Design review of the part built by this model. Coordinates are the model's own, in mm. A direction names the side the tool comes from. Coordinates: 2 decimals unless noted, no trailing zeros. Loops run counter-clockwise (first coordinate to the right, second up) from the corner with the lowest first, then second, coordinate; pieces in that order, holes last. Notation, with made-up numbers: (-3.75, -32.5) - (48.25, -32.5) arc R4 ccw to (48.25, -25.5) - close; hole circle Ø6 at (30, -12). An arc over 180 degrees is marked (long way). Use one line per item in the form item = value. Start each with the question number.
(1) Add section B-B (y = 11.75). State the section outline as (x, z) points.
(2) Clearance check with flat-ended pins moving along their axes: pin 1 Ø1.5 at (x, z) = (19.5, 19) entering from +Y; pin 2 Ø1 at (x, z) = (39, 16) entering from +Y. State where each tip first meets the part, or that it passes through.
(3) Add section D-D (z = 18.5). State the section outline as (x, y) points.
(4) The part is to be moulded in two halves that separate along Z. For faces 1 (the face through (-1, 0, -21)), 2 (the face through (-28, 2, 0)), say which applies: pulls with the +Z half, pulls with the -Z half, needs draft (parallel to the pull), parting line crosses it, or undercut.
(5) Add section A-A (z = 0). State the section outline as (x, y) points.
(6) Tool access review of faces 3 (the face through (-22, 2, 0)), 4 (the face through (-56, 14, -44)), 5 (the face through (57, 4, -43)): name each direction out of +Z, -Z, +X, -X, +Y, -Y from which nothing blocks a thin tool from reaching the whole face with its end or side.
(7) Add section C-C (x = 25). State the section outline as (y, z) points.
(8) For L1, parallel to X at y = 5.5, z = 18.5; L2, parallel to X at y = 2.25, z = 0; L3, parallel to Z at x = 56, y = 2.8, list the stretches that pass through material, from the lowest coordinate up.
```python
from build123d import *
from build123d.topology import SkipClean

# Parameters (mm, degrees)
SKETCH1_W               = 31
SKETCH1_H               = 26
SKETCH1_R               = 2.5
SKETCH1_R_2             = 5
BOSS_EXTRUDE1_DEPTH     = 4
FILLET1_R               = 4
BOSS_EXTRUDE2_START     = 10
SKETCH2_R               = 4
BOSS_EXTRUDE2_DEPTH     = 10
MIRROR2_START           = 10
MIRROR2_COPY_1_SKETCH_R = 4
MIRROR2_COPY_1_DEPTH    = 10
SKETCH3_R               = 1.75
CUT_EXTRUDE1_DEPTH      = 4
MIRROR4_COPY_1_SKETCH_R = 1.75
MIRROR4_COPY_1_DEPTH    = 4
SKETCH4_R               = 2.5
BOSS_EXTRUDE3_DEPTH     = 4
SKETCH5_R               = 1.75
CUT_EXTRUDE2_DEPTH      = 10
MIRROR6_COPY_1_SKETCH_R = 1.75
MIRROR6_COPY_1_DEPTH    = 10
CUT_EXTRUDE3_DEPTH      = 10


with BuildPart() as part:
    # Sketch1 → Boss-Extrude1 (new body)
    # profile 1 of 3: a face of its own
    with BuildSketch(Plane(origin=(0, 0, 0), x_dir=(1, 0, 0), z_dir=(0, 1, 0))):
        Polygon((-60, -13), (-60, -45), (60, -45), (60, -13), (29, -13), (29, 13), (60, 13), (60, 45), (-60, 45), (-60, 13), (-29, 13), (-29, -13), align=None)
    # profile 2 of 3: a face of its own
    with BuildSketch(Plane(origin=(0, 0, 0), x_dir=(1, 0, 0), z_dir=(0, 1, 0))):
        with Locations((-44.5, 0)):
            Rectangle(SKETCH1_W, SKETCH1_H)
        with Locations(Location((-51.5, -8, 0), (0, 0, 270))):
            Circle(SKETCH1_R, mode=Mode.SUBTRACT)
        with Locations(Location((-37.5, -8, 0), (0, 0, 270))):
            Circle(SKETCH1_R, mode=Mode.SUBTRACT)
        with Locations(Location((-51.5, 8, 0), (0, 0, 270))):
            Circle(SKETCH1_R, mode=Mode.SUBTRACT)
        with Locations(Location((-44.5, 0, 0), (0, 0, 270))):
            Circle(SKETCH1_R_2, mode=Mode.SUBTRACT)
        with Locations(Location((-37.5, 8, 0), (0, 0, 270))):
            Circle(SKETCH1_R, mode=Mode.SUBTRACT)
    # profile 3 of 3: a face of its own
    with BuildSketch(Plane(origin=(0, 0, 0), x_dir=(1, 0, 0), z_dir=(0, 1, 0))):
        with Locations((44.5, 0)):
            Rectangle(SKETCH1_W, SKETCH1_H)
        with Locations(Location((37.5, -8, 0), (0, 0, 270))):
            Circle(SKETCH1_R, mode=Mode.SUBTRACT)
        with Locations(Location((51.5, -8, 0), (0, 0, 270))):
            Circle(SKETCH1_R, mode=Mode.SUBTRACT)
        with Locations(Location((44.5, 0, 0), (0, 0, 270))):
            Circle(SKETCH1_R_2, mode=Mode.SUBTRACT)
        with Locations(Location((37.5, 8, 0), (0, 0, 270))):
            Circle(SKETCH1_R, mode=Mode.SUBTRACT)
        with Locations(Location((51.5, 8, 0), (0, 0, 270))):
            Circle(SKETCH1_R, mode=Mode.SUBTRACT)
    extrude(amount=BOSS_EXTRUDE1_DEPTH)

    # Fillet1
    fillet1_edges = [part.edges().sort_by_distance(p)[0] for p in [
        (-60, 2, -45),
        (60, 2, -45),
        (60, 2, 45),
        (-60, 2, 45),
    ]]
    fillet(fillet1_edges, radius=FILLET1_R)

    # Sketch2 → Boss-Extrude2 (add)
    with SkipClean():  # the faces are left unmerged after this step: merging them gives an invalid solid
        with BuildSketch(Plane(origin=(0, 4, 0), x_dir=(1, 0, 0), z_dir=(0, 1, 0)).offset(BOSS_EXTRUDE2_START)):
            with Locations(Location((-56, 41, 0), (0, 0, 90))):
                Circle(SKETCH2_R)
            Polygon((-53.1, 41), (-54.55, 43.511473671), (-57.45, 43.511473671), (-58.9, 41), (-57.45, 38.488526329), (-54.55, 38.488526329), align=None, mode=Mode.SUBTRACT)
        boss_extrude2 = extrude(amount=-BOSS_EXTRUDE2_DEPTH)

    # Mirror1: Boss-Extrude2 across plane
    add(boss_extrude2.mirror(Plane.XY))

    # Mirror2: Boss-Extrude2 across plane
    add(boss_extrude2.mirror(Plane(origin=(0, 0, 0), x_dir=(0, 0, 1), z_dir=(1, 0, 0))))

    # Mirror2 copy 1 sketch → Mirror2 copy 1 (add)
    with SkipClean():  # the faces are left unmerged after this step: merging them gives an invalid solid
        with BuildSketch(Plane(origin=(0, 4, 0), x_dir=(-1, 0, 0), z_dir=(0, 1, 0)).offset(MIRROR2_START)):
            with Locations(Location((-56, 41, 0), (0, 0, 90))):
                Circle(MIRROR2_COPY_1_SKETCH_R)
            Polygon((-53.1, 41), (-54.55, 43.511473671), (-57.45, 43.511473671), (-58.9, 41), (-57.45, 38.488526329), (-54.55, 38.488526329), align=None, mode=Mode.SUBTRACT)
        extrude(amount=-MIRROR2_COPY_1_DEPTH)

    # Sketch3 → Cut-Extrude1 (cut)
    with SkipClean():  # the faces are left unmerged after this step: merging them gives an invalid solid
        with BuildSketch(Plane(origin=(0, 4, 0), x_dir=(1, 0, 0), z_dir=(0, 1, 0))):
            with Locations(Location((-56, 41, 0), (0, 0, 270))):
                Circle(SKETCH3_R)
        cut_extrude1 = extrude(amount=-CUT_EXTRUDE1_DEPTH, mode=Mode.SUBTRACT)

    # Mirror3: Cut-Extrude1 across plane
    with SkipClean():  # the faces are left unmerged after this step: merging them gives an invalid solid
        add(cut_extrude1.mirror(Plane(origin=(0, 0, 0), x_dir=(0, 0, 1), z_dir=(1, 0, 0))), mode=Mode.SUBTRACT)

    # Mirror4: Cut-Extrude1 across plane
    with SkipClean():  # the faces are left unmerged after this step: merging them gives an invalid solid
        add(cut_extrude1.mirror(Plane.XY), mode=Mode.SUBTRACT)

    # Mirror4 copy 1 sketch → Mirror4 copy 1 (cut)
    with SkipClean():  # the faces are left unmerged after this step: merging them gives an invalid solid
        with BuildSketch(Plane(origin=(0, 4, 0), x_dir=(-1, 0, 0), z_dir=(0, 1, 0))):
            with Locations(Location((-56, 41, 0), (0, 0, 270))):
                Circle(MIRROR4_COPY_1_SKETCH_R)
        extrude(amount=-MIRROR4_COPY_1_DEPTH, mode=Mode.SUBTRACT)

    # Sketch4 → Boss-Extrude3 (add)
    with SkipClean():  # the faces are left unmerged after this step: merging them gives an invalid solid
        with BuildSketch(Plane(origin=(0, 4, 0), x_dir=(1, 0, 0), z_dir=(0, 1, 0))):
            with Locations(Location((-18.5, 18.5, 0), (0, 0, 270))):
                Circle(SKETCH4_R)
            with Locations(Location((18.5, 18.5, 0), (0, 0, 90))):
                Circle(SKETCH4_R)
            with Locations(Location((18.5, -18.5, 0), (0, 0, 270))):
                Circle(SKETCH4_R)
            with Locations(Location((-18.5, -18.5, 0), (0, 0, 90))):
                Circle(SKETCH4_R)
        extrude(amount=BOSS_EXTRUDE3_DEPTH)

    # Sketch5 → Cut-Extrude2 (cut)
    with SkipClean():  # the faces are left unmerged after this step: merging them gives an invalid solid
        with BuildSketch(Plane(origin=(0, 8, 0), x_dir=(1, 0, 0), z_dir=(0, 1, 0))):
            with Locations(Location((-18.5, 18.5, 0), (0, 0, 270))):
                Circle(SKETCH5_R)
        cut_extrude2 = extrude(amount=-CUT_EXTRUDE2_DEPTH, mode=Mode.SUBTRACT)

    # Mirror5: Cut-Extrude2 across plane
    with SkipClean():  # the faces are left unmerged after this step: merging them gives an invalid solid
        add(cut_extrude2.mirror(Plane(origin=(0, 0, 0), x_dir=(0, 0, 1), z_dir=(1, 0, 0))), mode=Mode.SUBTRACT)

    # Mirror6: Cut-Extrude2 across plane
    with SkipClean():  # the faces are left unmerged after this step: merging them gives an invalid solid
        add(cut_extrude2.mirror(Plane.XY), mode=Mode.SUBTRACT)

    # Mirror6 copy 1 sketch → Mirror6 copy 1 (cut)
    with SkipClean():  # the faces are left unmerged after this step: merging them gives an invalid solid
        with BuildSketch(Plane(origin=(0, 8, 0), x_dir=(-1, 0, 0), z_dir=(0, 1, 0))):
            with Locations(Location((-18.5, 18.5, 0), (0, 0, 270))):
                Circle(MIRROR6_COPY_1_SKETCH_R)
        extrude(amount=-MIRROR6_COPY_1_DEPTH, mode=Mode.SUBTRACT)

    # Sketch6 → Cut-Extrude3 (cut)
    with SkipClean():  # the faces are left unmerged after this step: merging them gives an invalid solid
        with BuildSketch(Plane(origin=(0, 4, 0), x_dir=(1, 0, 0), z_dir=(0, 1, 0))):
            with BuildLine():
                Line((-12, -15), (12, -15))
                ThreePointArc((12, -15), (14.121320344, -14.121320344), (15, -12))
                Line((15, -12), (15, 12))
                ThreePointArc((15, 12), (14.121320344, 14.121320344), (12, 15))
                Line((12, 15), (-12, 15))
                ThreePointArc((-12, 15), (-14.121320344, 14.121320344), (-15, 12))
                Line((-15, 12), (-15, -12))
                ThreePointArc((-15, -12), (-14.121320344, -14.121320344), (-12, -15))
            make_face()
            with BuildLine():
                Line((-28, -7.5), (-28, 7.5))
                ThreePointArc((-28, 7.5), (-25, 10.5), (-22, 7.5))
                Line((-22, 7.5), (-22, -7.5))
                ThreePointArc((-22, -7.5), (-25, -10.5), (-28, -7.5))
            make_face()
            with BuildLine():
                Line((28, -7.5), (28, 7.5))
                ThreePointArc((28, 7.5), (25, 10.5), (22, 7.5))
                Line((22, 7.5), (22, -7.5))
                ThreePointArc((22, -7.5), (25, -10.5), (28, -7.5))
            make_face()
            with BuildLine():
                Line((-40, 38), (40, 38))
                ThreePointArc((40, 38), (43, 35), (40, 32))
                Line((40, 32), (-40, 32))
                ThreePointArc((-40, 32), (-43, 35), (-40, 38))
            make_face()
            with BuildLine():
                Line((-40, -38), (40, -38))
                ThreePointArc((40, -38), (43, -35), (40, -32))
                Line((40, -32), (-40, -32))
                ThreePointArc((-40, -32), (-43, -35), (-40, -38))
            make_face()
        extrude(amount=-CUT_EXTRUDE3_DEPTH, mode=Mode.SUBTRACT)


solid = part.part
```
Computed values:
q1.outline = circle Ø8 at (-56, -41); circle Ø8 at (-56, 41); circle Ø8 at (56, -41); circle Ø8 at (56, 41); hole (-58.9, -41) - (-57.45, -43.51) - (-54.55, -43.51) - (-53.1, -41) - (-54.55, -38.49) - (-57.45, -38.49) - close; hole (-58.9, 41) - (-57.45, 38.49) - (-54.55, 38.49) - (-53.1, 41) - (-54.55, 43.51) - (-57.45, 43.51) - close; hole (53.1, -41) - (54.55, -43.51) - (57.45, -43.51) - (58.9, -41) - (57.45, -38.49) - (54.55, -38.49) - close; hole (53.1, 41) - (54.55, 38.49) - (57.45, 38.49) - (58.9, 41) - (57.45, 43.51) - (54.55, 43.51) - close
q2.pin_1 = 8
q2.pin_2 = 4
q3.outline = (-60, 0) - (-20.25, 0) - (-20.25, 8) - (-21, 8) - (-21, 4) - (-60, 4) - close; (-16.75, 0) - (16.75, 0) - (16.75, 8) - (16, 8) - (16, 4) - (-16, 4) - (-16, 8) - (-16.75, 8) - close; (20.25, 0) - (60, 0) - (60, 4) - (21, 4) - (21, 8) - (20.25, 8) - close
q4.face_1 = needs draft
q4.face_2 = undercut
q5.outline = (-60, 0) - (-49.5, 0) - (-49.5, 4) - (-60, 4) - close; (-39.5, 0) - (-28, 0) - (-28, 4) - (-39.5, 4) - close; (-22, 0) - (-15, 0) - (-15, 4) - (-22, 4) - close; (15, 0) - (22, 0) - (22, 4) - (15, 4) - close; (28, 0) - (39.5, 0) - (39.5, 4) - (28, 4) - close; (49.5, 0) - (60, 0) - (60, 4) - (49.5, 4) - close
q6.face_3 = +Y, -Y
q6.face_4 = +Z, -Z, +X, -X, +Y
q6.face_5 = +Y
q7.outline = (0, -45) - (4, -45) - (4, -38) - (0, -38) - close; (0, -32) - (4, -32) - (4, -10.5) - (0, -10.5) - close; (0, 10.5) - (4, 10.5) - (4, 32) - (0, 32) - close; (0, 38) - (4, 38) - (4, 45) - (0, 45) - close
q8.L1 = -21 to -20.25, -16.75 to -16, 16 to 16.75, 20.25 to 21
q8.L2 = -60 to -49.5, -39.5 to -28, -22 to -15, 15 to 22, 28 to 39.5, 49.5 to 60
q8.L3 = -45 to -42.75, -39.25 to 39.25, 42.75 to 45
